Autodesk Inventor part; units mm, degrees
ref_plane "YZ Plane" through (0, 0, 0) normal (1, 0, 0) x (0, 1, 0)
ref_plane "XZ Plane" through (0, 0, 0) normal (0, 1, 0) x (-1, 0, 0)
ref_plane "XY Plane" through (0, 0, 0) normal (0, 0, 1) x (1, 0, 0)
sketch "Sketch1" plane through (0, 0, 0) normal (0, 1, 0) x (-1, 0, 0)
  circle A0 centre (0, 0) radius 26
  dimension "d0" = 52
extrude "Extrusion1" add sketch "Sketch1" along normal blind 7.6
chamfer "Chamfer2" distance 2 angle 45 1 edges at (26, 0, 0)
sketch "Sketch2" plane through (0, 7.6, 0) normal (0, 1, 0) x (1, 0, 0)
  line L0 (-12.6, -9.19) -> (23.96, -9.19)
  line L1 (23.96, -9.19) -> (23.96, 9.19)
  line L2 (23.96, 9.19) -> (-12.6, 9.19)
  line L3 (-12.6, 9.19) -> (-12.6, -9.19)
  point P0 (0, 0)
  dimension "d5" = 36.56
  dimension "d6" = 18.38
  dimension "d7" = 9.19
  dimension "d8" = 12.6
extrude "Extrusion2" cut sketch "Sketch2" against normal blind 5
sketch "Sketch3" plane through (23.96, 7.6, -9.19) normal (-1, 0, 0) x (0, 0, 1)
  line L0 (3.6, 0) -> (14.78, 0)
  line L1 (14.78, 0) -> (14.78, -3.6)
  line L2 (14.78, -3.6) -> (3.6, -3.6)
  line L3 (3.6, -3.6) -> (3.6, 0)
  line L4 (0, 0) -> (18.38, 0)
  line L5 (0, -5) -> (18.38, -5)
  line L6 (0, 0) -> (0, -5)
  line L7 (18.38, 0) -> (18.38, -5)
  point P0 (9.19, -7.6)
  dimension "d11" = 0
  dimension "d14" = 3.6
  dimension "d44" = 3.6
  dimension "d47" = 1.4
extrude "Extrusion3" cut sketch "Sketch3" against normal through all contours L0 L1 L2 L3
ref_plane "Work Plane1" through (-12.6, 7.6, 0) normal (0, 0, 1) x (1, 0, 0)
sketch "Sketch7" plane through (0, 2.6, 0) normal (0, 1, 0) x (1, 0, 0)
  line L0 (-12.6, 6.35) -> (22.96, 6.35)
  line L1 (22.96, 6.35) -> (22.96, -6.35)
  line L2 (22.96, -6.35) -> (-12.6, -6.35)
  line L3 (-12.6, -6.35) -> (-12.6, 6.35)
  line L4 (36.4, 0) -> (-36.4, 0)
  line L5 (-12.6, -9.19) -> (-12.6, 9.19)
  point P0 (0, 0)
  dimension "d28" = 12.7
  dimension "d29" = 35.56
  dimension "d30" = 6.35
  dimension "d31" = 0
extrude "Extrusion5" cut sketch "Sketch7" against normal blind 1.6
sketch "Sketch4" plane through (0, 7.6, 0) normal (0, 1, 0) x (1, 0, 0)
  circle A0 centre (-21, 0) radius 2.8
  arc A1 (25.392, 5.59) -> (25.392, -5.59) centre (0, 0) ccw
  point P0 (24.6995, 8.12)
  point P1 (24.6995, -8.12)
  dimension "d17" = 5.6
  dimension "d23" = 21
extrude "Extrusion4" cut sketch "Sketch4" against normal blind 5.2
fillet "Fillet4" radius 1.6 1 edges at (-23.8, 7.6, 0)
pattern_circular "Circular Pattern2" count 5 over 240 about axis through (0, 7.6, 0) along (0, 1, 0) of "Extrusion4", "Fillet4" both ways yes
chamfer "Chamfer3" distance 1.5 distance2 5 1 edges at (-12.6, 1, 0) measured on face at (-12.6, 5.9333, -2.1167)
equation "\"d44\" = d14"
equation "\"d30\" = 0.5 * d28"
equation "\"d24\" = 0.5 * d6"
properties part number "_3DPrint"
Work out the finished part from the listing and answer in its coordinate system (mm). A direction names the side the tool comes from. Give positions to 0.01 mm unless a question says otherwise; leave off trailing zeros. Write each loop counter-clockwise with the first axis right and the second up, starting at its lowest first coordinate (ties: lowest second). Pieces come first, ordered by that corner, then holes.
(1) Which of the six approach directions +Z, -Z, +X, -X, +Y, -Y give full straight-line access (tool end or side, diameter ignored) to faces 4 (the flat face through (-10.07, 1.74, -0.09)), 5 (the flat face through (25, 6, -5.59)), 6 (the flat face through (0, 0, 0))?
Final values:
face 4: +Y
face 5: +X, +Y
face 6: +Z, -Z, +X, -X, -Y
(2) The mould has two halves that part along X. Classify faces 1 (the flat face through (-10, 2.4, -18)), 2 (the flat face through (25, 6, 5.59)), 3 (the flat face through (5, 5, 9.19)): pulls with the +X half, pulls with the -X half, needs draft (parallel to the pull), parting line crosses it, or undercut.
Final values:
face 1: undercut
face 2: needs draft
face 3: undercut
(3) Flat-ended cylindrical pins translate along their axes: pin 1 Ø2.5 at (y, z) = (6, 4) entering from -X; pin 2 Ø2 at (x, z) = (25.5, 0.5) entering from +Y; pin 3 Ø5 at (x, z) = (-3.5, 14) entering from -Y; pin 4 Ø4 at (x, y) = (11.5, 3) entering from -Z. Find the tip coordinate at first contact, or state that the pin passes through.
Final values:
pin 1: stops at x = -25.85
pin 2: stops at y = 4
pin 3: stops at y = 0
pin 4: stops at z = -24.2
(4) The part is cut by section B-B on z = 0. Write down the section's boundary in (x, y), plus the area to 3 significant figures.
Final values:
outline: (-26, 2) - (-24, 0) - (24, 0) - (26, 2) - (26, 4) - (23.96, 4) - (23.96, 2.6) - (22.96, 2.6) - (22.96, 1) - (-7.6, 1) - (-12.6, 2.5) - (-12.6, 7.6) - (-16.6, 7.6) arc R1.6 ccw to (-18.2, 6) - (-18.2, 2.4) - (-23.8, 2.4) - (-23.8, 6) arc R1.6 ccw to (-25.4, 7.6) - (-26, 7.6) - close
area: 118 mm2
(5) The part is cut by section A-A on x = 0. Write down the section's boundary in (y, z).
Final values:
outline: (0, -24) - (2, -26) - (7.6, -26) - (7.6, -9.19) - (2.6, -9.19) - (2.6, -6.35) - (1, -6.35) - (1, 6.35) - (2.6, 6.35) - (2.6, 9.19) - (7.6, 9.19) - (7.6, 26) - (2, 26) - (0, 24) - close
(6) Straight lines are drawn through the part: line 1 (Z direction, x = -13, y = 3.75); line 2 (Z direction, x = 10.5, y = 5.1); line 3 (Z direction, x = 8, y = 6). For each, find the intervals that lie inside material, in ascending order.
Final values:
line 1: z = -22.52 to -19.45, -16.93 to 16.93, 19.45 to 22.52
line 2: z = -23.79 to -20.99, -15.39 to -9.19, 9.19 to 15.39, 20.99 to 23.79
line 3: z = -24.74 to -19.45, -16.93 to -9.19, 9.19 to 16.93, 19.45 to 24.74
